The drawing under review shows one solid part. Ordinate dimensions are in mm from its lowest x, y, z. Round coordinates to 2 decimals unless told otherwise and drop trailing zeros. Write each loop counter-clockwise with the first axis right and the second up, starting at its lowest first coordinate (ties: lowest second). Pieces come first, ordered by that corner, then holes. Notation, with made-up numbers: (8, 24.25) -> (27, 24.25) arc R20 cw to (27, 49.25) -> close; hole circle Ø2 at (-14, 57). An arc over 180 degrees is marked (long way). Write item = value, one per line. Start each with the question number.
Item 1: Add section B-B, the plane y = 35. State the section outline as (x, z) points.
Item 2: To check wall thickness, follow L1, parallel to Y at x = 50, z = 32.4; L2, parallel to Y at x = 50, z = 8; L3, parallel to X at y = 36.5, z = 30.5. State the ranges of each line that lie inside material, in increasing order.
Item 3: Mouldability with a two-part tool opening along Y and no side actions: class the marked faces 1, 2 and 3 as released by +Y, released by -Y, zero draft, split by the parting line, or undercut.
Item 4: For pin 1 Ø6 at (x, y) = (47.5, 36.5) entering from +Z, flat-tipped, find the tip position at first contact; note if it passes through.
Item 5: Add section A-A, the plane x = 50. State the section outline as (y, z) points, then the cut area to 3 significant figures.
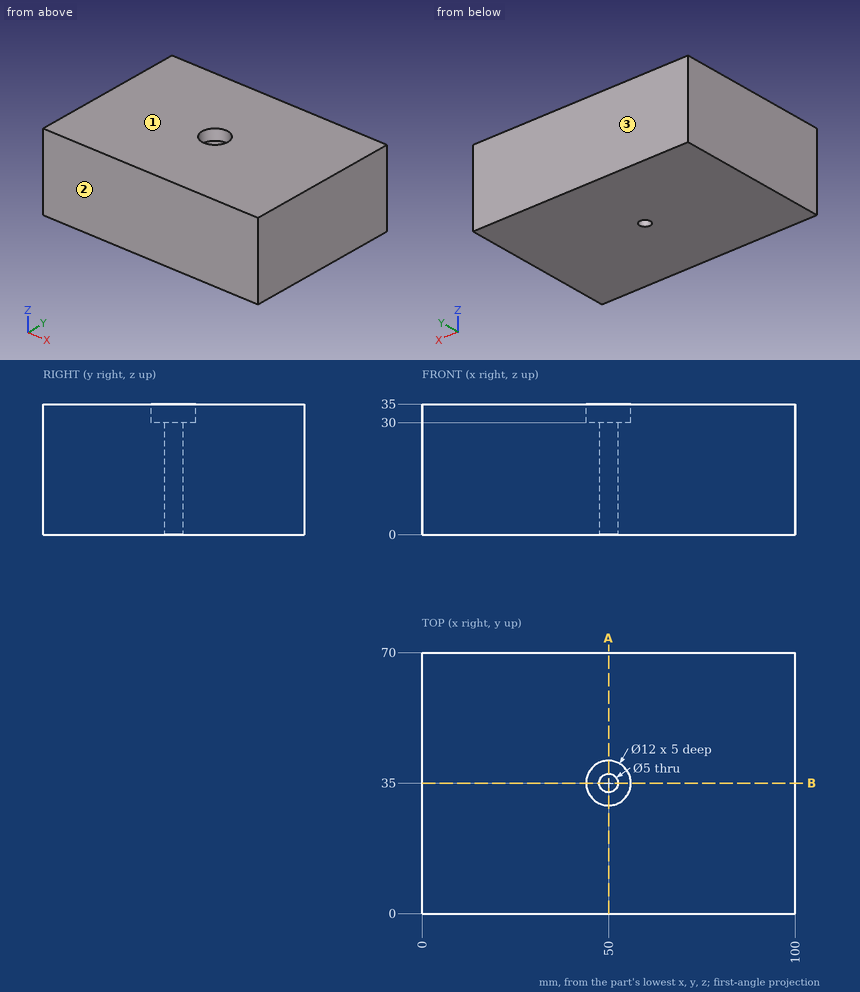
Result set:
q1.outline = (0, 0) -> (47.5, 0) -> (47.5, 30) -> (44, 30) -> (44, 35) -> (0, 35) -> close; (52.5, 0) -> (100, 0) -> (100, 35) -> (56, 35) -> (56, 30) -> (52.5, 30) -> close
q2.L1 = 0 to 29, 41 to 70
q2.L2 = 0 to 32.5, 37.5 to 70
q2.L3 = 0 to 44.19, 55.81 to 100
q3.face_1 = zero draft
q3.face_2 = released by -Y
q3.face_3 = released by +Y
q4.pin_1 = 30
q5.outline = (0, 0) -> (32.5, 0) -> (32.5, 30) -> (29, 30) -> (29, 35) -> (0, 35) -> close; (37.5, 0) -> (70, 0) -> (70, 35) -> (41, 35) -> (41, 30) -> (37.5, 30) -> close
q5.area = 2,240 mm²
